Input: part model. Units: mm. Frame: model coordinates. A direction names the side the tool comes from. Coordinates: 2 decimals unless noted, no trailing zeros. Order: outer loops, then holes, each group sorted by start corner. A loop starts at its lowest first (then second) coordinate and runs counter-clockwise, first axis right, second up. Notation, with made-up numbers: (-36.5, 4) - (-15.5, 4) arc R19 ccw to (-15.5, 31) - close; hole circle Ø10 at (36, 69.25). An arc over 180 degrees is marked (long way). One line per question, with ' | ' between items. Start each with the question number.
```python
from build123d import *

# Parameters (mm, degrees)
F0_R     = 1.7526
F0_W     = 38.1
F0_H     = 12.7
F1_DEPTH = 3.0988
F2_R     = 3.175


with BuildPart() as f1:
    # F0 (on Top) → F1 (new body)
    with BuildSketch(Plane.XY):
        Polygon((44.45, 88.9), (-44.45, 88.9), (-44.45, 82.55), (-47.5488, 82.55), (-47.5488, 69.85), (-44.45, 69.85), (-44.45, 39.8526), (-41.275, 39.8526), (-41.275, 42.06875), (-38.496875, 42.06875), (-38.496875, 39.8526), (-32.146875, 39.8526), (-32.146875, 36.3474), (-38.496875, 36.3474), (-38.496875, 34.13125), (-41.275, 34.13125), (-41.275, 36.3474), (-44.45, 36.3474), (-44.45, 6.35), (-47.5488, 6.35), (-47.5488, -6.35), (-44.45, -6.35), (-44.45, -36.3474), (-41.275, -36.3474), (-41.275, -34.13125), (-38.496875, -34.13125), (-38.496875, -36.3474), (-32.146875, -36.3474), (-32.146875, -39.8526), (-38.496875, -39.8526), (-38.496875, -42.06875), (-41.275, -42.06875), (-41.275, -39.8526), (-44.45, -39.8526), (-44.45, -69.85), (-47.5488, -69.85), (-47.5488, -82.55), (-44.45, -82.55), (-44.45, -88.9), (44.45, -88.9), (44.45, -82.55), (47.5488, -82.55), (47.5488, -69.85), (44.45, -69.85), (44.45, -39.8526), (41.275, -39.8526), (41.275, -42.06875), (38.496875, -42.06875), (38.496875, -39.8526), (32.146875, -39.8526), (32.146875, -36.3474), (38.496875, -36.3474), (38.496875, -34.13125), (41.275, -34.13125), (41.275, -36.3474), (44.45, -36.3474), (44.45, -6.35), (47.5488, -6.35), (47.5488, 6.35), (44.45, 6.35), (44.45, 36.3474), (41.275, 36.3474), (41.275, 34.13125), (38.496875, 34.13125), (38.496875, 36.3474), (32.146875, 36.3474), (32.146875, 39.8526), (38.496875, 39.8526), (38.496875, 42.06875), (41.275, 42.06875), (41.275, 39.8526), (44.45, 39.8526), (44.45, 69.85), (47.5488, 69.85), (47.5488, 82.55), (44.45, 82.55), align=None)
        with Locations((-20, -27.1526)):
            Circle(F0_R, mode=Mode.SUBTRACT)
        with Locations((0, -63.5)):
            Rectangle(F0_W, F0_H, mode=Mode.SUBTRACT)
        with Locations((20, -27.1526)):
            Circle(F0_R, mode=Mode.SUBTRACT)
        with Locations((0, 63.5)):
            Rectangle(F0_W, F0_H, mode=Mode.SUBTRACT)
    extrude(amount=F1_DEPTH)

    # F2
    f2_edges = [f1.edges().sort_by_distance(p)[0] for p in [
        (19.05, 57.15, 1.5494),
        (19.05, -69.85, 1.5494),
        (-19.05, 57.15, 1.5494),
        (-19.05, -69.85, 1.5494),
        (19.05, 69.85, 1.5494),
        (19.05, -57.15, 1.5494),
        (-19.05, -57.15, 1.5494),
        (-19.05, 69.85, 1.5494),
    ]]
    fillet(f2_edges, radius=F2_R)


solid = f1.part
```
(1) Section C-C (z = 1.65). State how many separate pieces and enclosed holes the cut face has, then the cut area to 3 significant figures.
(2) Section D-D (y = 55). Output: boundary loops of the cut face in (x, z), then the cut area to 3 significant figures.
(3) Section B-B (x = 6). Output: boundary loops of the cut face in (y, z).
(4) Draft query along X for faces 4 (the face through (43, 39.853, 2)), 5 (the face through (47.549, 76, 2)), 6 (the face through (0, 69.85, 2)). Return one class per face: +X half, -X half, draft (parallel to the pull), parting line (faces both ways), or undercut.
(5) Material intervals for line 1 along X through (y, z) = (-36, 2.35) (3 decimals); line 2 along Y through (x, z) = (43.5, 0.8); line 3 along Y through (x, z) = (-3, 1.85), sorted ascending. Write a range as from..to.
(6) Reachability of faces 1 (the face through (0, -57.15, 2)), 2 (the face through (44.45, 55, 2)), 3 (the face through (-46, -69.85, 2)) from +Z, -Z, +X, -X, +Y, -Y: full face, straight path, thin tool, end or side. Return the list, or none.
(7) Section A-A (x = -36). Output: boundary loops of the cut face in (y, z), then the cut area to 3 significant figures.
(8) Pin query (flat end, axial travel): pin 1 (0.9 mm diameter, centred on y = 37.5, z = 1, fed in from +X); pin 2 (1 mm diameter, centred on y = -41, z = 2, fed in from -X); pin 3 (1.5 mm diameter, centred on y = 37.5, z = 1, fed in from -X). Return the tip coordinate at first contact, or that it passes through.
Worked answers:
1) separate pieces: 1 | enclosed holes: 4 | area: 14,900 mm²
2) outline: (-44.45, 0) - (44.45, 0) - (44.45, 3.1) - (-44.45, 3.1) - close | area: 275 mm²
3) outline: (-88.9, 0) - (-69.85, 0) - (-69.85, 3.1) - (-88.9, 3.1) - close; (-57.15, 0) - (57.15, 0) - (57.15, 3.1) - (-57.15, 3.1) - close; (69.85, 0) - (88.9, 0) - (88.9, 3.1) - (69.85, 3.1) - close
4) face 4: draft | face 5: +X half | face 6: undercut
5) line 1: x = -44.45..-41.275, -38.497..38.497, 41.275..44.45 | line 2: y = -88.9..-39.85, -36.35..36.35, 39.85..88.9 | line 3: y = -88.9..-69.85, -57.15..57.15, 69.85..88.9
6) face 1: +Z, -Z | face 2: +Z, -Z, +X | face 3: +Z, -Z, -X
7) outline: (-88.9, 0) - (-39.85, 0) - (-39.85, 3.1) - (-88.9, 3.1) - close; (-36.35, 0) - (36.35, 0) - (36.35, 3.1) - (-36.35, 3.1) - close; (39.85, 0) - (88.9, 0) - (88.9, 3.1) - (39.85, 3.1) - close | area: 529 mm²
8) pin 1: stops at x = 32.15 | pin 2: stops at x = -44.45 | pin 3: stops at x = -32.15
